Input: part model. Units: mm. Frame: model coordinates. A direction names the side the tool comes from. Coordinates: 2 decimals unless noted, no trailing zeros. Write each loop counter-clockwise with the first axis right and the second up, starting at its lowest first coordinate (ties: lowest second). Pieces come first, ordered by that corner, then holes. Notation, with made-up numbers: M 61,-27.75 L 104,-27.75 A28 cw 104,4.25 Z; hole C 57.5,87 d4. An arc over 180 degrees is marked long. Use one line per item in the form item = value.
from build123d import *

# Parameters (mm, degrees)
BOSS_EXTRUDE1_DEPTH = 5
SKETCH2_OUTSIDE_W   = 44.609
SKETCH2_OUTSIDE_H   = 67.511
CUT_EXTRUDE1_DEPTH  = 5
SKETCH3_W           = 5
SKETCH3_H           = 5
BOSS_EXTRUDE2_DEPTH = 5


with BuildPart() as part:
    # Sketch1 → Boss-Extrude1 (new body)
    with BuildSketch(Plane.XY):
        with BuildLine():
            Line((-20, 0), (0, 0))
            Line((0, 0), (-27.704916794, 53.220649991))
            ThreePointArc((-27.704916794, 53.220649991), (-29.652591379, 25.770621947), (-20, 0))
        make_face()
    extrude(amount=BOSS_EXTRUDE1_DEPTH)

    # Sketch2 outside → Cut-Extrude1 (cut)
    with BuildSketch(Plane.XY.offset(5)):
        with Locations((-15.1595, 26.6105)):
            Rectangle(SKETCH2_OUTSIDE_W, SKETCH2_OUTSIDE_H)
        with BuildLine():
            Line((-12, 4.5), (-12, 7))
            Line((-12, 7), (-9, 7))
            Line((-9, 7), (-9, 4.5))
            Line((-9, 4.5), (-7.75, 4.5))
            Line((-7.75, 4.5), (-7.75, 2.5))
            Line((-7.75, 2.5), (-9, 2.5))
            Line((-9, 2.5), (-9, 0))
            Line((-9, 0), (0, 0))
            Line((0, 0), (-7.387977812, 14.192173331))
            Line((-7.387977812, 14.192173331), (-9.605504895, 13.037801798))
            Line((-9.605504895, 13.037801798), (-9.028319128, 11.929038256))
            Line((-9.028319128, 11.929038256), (-10.802340795, 11.00554103))
            Line((-10.802340795, 11.00554103), (-11.379526561, 12.114304571))
            Line((-11.379526561, 12.114304571), (-13.597053644, 10.959933038))
            Line((-13.597053644, 10.959933038), (-14.982299484, 13.620965538))
            Line((-14.982299484, 13.620965538), (-12.764772401, 14.775337071))
            Line((-12.764772401, 14.775337071), (-13.341958167, 15.884100612))
            Line((-13.341958167, 15.884100612), (-11.567936501, 16.807597839))
            Line((-11.567936501, 16.807597839), (-10.990750734, 15.698834297))
            Line((-10.990750734, 15.698834297), (-8.773223651, 16.85320583))
            Line((-8.773223651, 16.85320583), (-18.931693143, 36.36744416))
            Line((-18.931693143, 36.36744416), (-21.149220226, 35.213072627))
            Line((-21.149220226, 35.213072627), (-20.572034459, 34.104309086))
            Line((-20.572034459, 34.104309086), (-22.346056125, 33.180811859))
            Line((-22.346056125, 33.180811859), (-22.923241892, 34.289575401))
            Line((-22.923241892, 34.289575401), (-25.140768975, 33.135203868))
            Line((-25.140768975, 33.135203868), (-26.526014815, 35.796236367))
            Line((-26.526014815, 35.796236367), (-24.308487732, 36.9506079))
            Line((-24.308487732, 36.9506079), (-24.885673498, 38.059371442))
            Line((-24.885673498, 38.059371442), (-23.111651832, 38.982868668))
            Line((-23.111651832, 38.982868668), (-22.534466065, 37.874105127))
            Line((-22.534466065, 37.874105127), (-20.316938982, 39.02847666))
            Line((-20.316938982, 39.02847666), (-27.704916794, 53.220649991))
            ThreePointArc((-27.704916794, 53.220649991), (-29.652591379, 25.770621947), (-20, 0))
            Line((-20, 0), (-12, 0))
            Line((-12, 0), (-12, 2.5))
            Line((-12, 2.5), (-13.25, 2.5))
            Line((-13.25, 2.5), (-13.25, 4.5))
            Line((-13.25, 4.5), (-12, 4.5))
        make_face(mode=Mode.SUBTRACT)
    extrude(amount=-CUT_EXTRUDE1_DEPTH, mode=Mode.SUBTRACT)

    # Sketch3 → Boss-Extrude2 (add)
    with BuildSketch(Plane.XY.offset(5)):
        Polygon((-23.269862628, 55.529393057), (-27.704916794, 53.220649991), (-22.625682049, 43.463530826), (-18.190627883, 45.772273892), align=None)
        Polygon((-12.187895911, 34.241133061), (-16.622950076, 31.932389994), (-11.081966718, 21.288259996), (-6.646912552, 23.597003062), align=None)
        Polygon((-5.079234746, 9.757119165), (0, 0), (-4, 0), (-4, -5), (5.636909734, -5), (5.636909734, 0), (-0.64418058, 12.065862231), align=None)
        with Locations((-17.5, -2.5)):
            Rectangle(SKETCH3_W, SKETCH3_H)
    extrude(amount=-BOSS_EXTRUDE2_DEPTH)


solid = part.part
(1) Pull-direction query (Y, two-part tool) for faces 1 (the flat face through (-11, 7, 3)), 2 (the flat face through (-14.374, 33.103, 2.535)), 3 (the flat face through (-9.903, 11.474, 2.535)); classes: pulls with the +Y half, pulls with the -Y half, needs draft (parallel to the pull), parting line crosses it, or undercut.
Computed:
face_1 = pulls with the -Y half
face_2 = pulls with the +Y half
face_3 = undercut
(2) Set-up query: faces 4 (the flat face through (-20, -3, 3)), 5 (the flat face through (-7, 0, 2)), 6 (the flat face through (-8.481, 13.623, 2.535)), 7 (the flat face through (-21.455, 41.215, 2.465)). Return all of +Z, -Z, +X, -X, +Y, -Y with unobstructed straight access to the full face (end or side cutting, diameter ignored); none if empty.
Computed:
face_4 = +Z, -Z, -X, -Y
face_5 = +Z, -Z, -Y
face_6 = +Z, -Z
face_7 = +Z, -Z, +X
(3) First-contact query: pin 1 Ø0.6 at (x, z) = (-12.5, 3.5) entering from -Y; pin 2 Ø1.2 at (y, z) = (1.5, 3.5) entering from -X; pin 3 Ø0.6 at (x, z) = (-8.5, 3) entering from +Y. Flat tips, straight axial feed; report the tip coordinate or a pass-through.
Computed:
pin_1 = 0
pin_2 = -21.3
pin_3 = 27.73
(4) Section query B-B on x = 3.5. Return the cut outline in (y, z), plus the area to 3 significant figures.
Computed:
outline = M -5,0 L 4.1,0 L 4.1,5 L -5,5 Z
area = 45.5 mm^2
(5) Section query A-A on y = 18. Return the cut outline in (x, z) (3 decimals), plus the area to 3 significant figures.
Computed:
outline = M -28.035,0 L -9.37,0 L -9.37,5 L -28.035,5 Z
area = 93.3 mm^2
(6) Line query: probe 1 along X at (y, z) = (-1, 3.45); probe 2 along Y at (x, z) = (-10, 3.05); probe 3 along Y at (x, z) = (-21, 4.25). Output: solid intervals per line, ascending.
Computed:
probe_1 = -20 to -15, -4 to 5.64
probe_2 = 7 to 11.42, 16.21 to 19.21, 21.85 to 30.04
probe_3 = 1.6 to 33.88, 34.93 to 35.29, 38.67 to 40.34, 44.31 to 51.17
